Build history of the part. All positions in model axes, mm. A direction names the side the tool comes from. Give positions to 0.01 mm unless a question says otherwise; leave off trailing zeros. Loops run counter-clockwise (first coordinate to the right, second up) from the corner with the lowest first, then second, coordinate; pieces in that order, holes last.
1) Band-saw the part on C-C on y = 13.5. List the corners of the cut face in (x, z).
2) Band-saw the part on B-B on x = 1.5. List the corners of the cut face in (y, z).
3) Band-saw the part on D-D on z = 4.5. List the corners of the cut face in (x, y), then the cut area to 3 significant figures.
4) 3-axis set-ups, long thin cutter, end or side, ignore diameter. For faces 1 (the flat face through (3.81, 32.6, 6.4)), 2 (the flat face through (-3.81, 25, 6)), 3 (the flat face through (-0.1, 26.386, -3.5)): which of +Z, -Z, +X, -X, +Y, -Y reach the whole face in a straight line?
5) Band-saw the part on A-A on z = 9. List the corners of the cut face in (x, y).
6) Flat gauge pins, fed straight in: P1, Ø1, axis at y = 33, z = -5, coming from the -X side; P2, Ø6, axis at y = 6.5, z = 6.5, coming from the +X side; P3, Ø2, axis at x = 1.5, y = 27, coming from the +Z side. Where does each tip first touch, or does it go through?
7) Two-plate mould, pull along Z, no slides. Class faces 4 (the flat face through (0.04, 32.11, -5.47)), 5 (the flat face through (-2.54, 33, -5)), 6 (the cylindrical face through (-0.417, 15.653, 3.173)): +Z half, -Z half, draft (parallel to the pull), parting line (faces both ways), or undercut.
8) Wall check: line 1 (Y direction, x = 2.25, z = 4.5); line 2 (Z direction, x = 0, y = 13); line 3 (X direction, y = 11.5, z = 0). Give the ranges that are in metal, low to high.
```python
from build123d import *

# Parameters (mm, degrees)
F1_R          = 5
F2_DEPTH      = 34.64052
F3_W          = 5.08
F3_H          = 2.89434
F4_DEPTH      = 34.64052
F6_W          = 10.16
F6_H          = 5.08
F7_DEPTH      = 25.4
F8_W          = 2.54
F8_H          = 7.62
F9_DEPTH      = 3.81
F9_DEPTH_BACK = 3.81
F5_R          = 3.2004
F10_DEPTH     = 31.75
F11_R         = 0.762
F12_SIZE      = 1.27
F13_R         = 0.508


with BuildPart() as f2:
    # F1 (on Front) → F2 (new body)
    with BuildSketch(Plane.XZ):
        Circle(F1_R)
    extrude(amount=-F2_DEPTH)

    # F3 (on face) → F4 (join, through all)
    with BuildSketch(Plane.XZ):
        with Locations((0, -4.64757)):
            Rectangle(F3_W, F3_H)
    extrude(amount=-F4_DEPTH)

    # F6 (on Top) → F7 (cut)
    with BuildSketch(Plane.XY):
        with Locations((0, 28.92552)):
            Rectangle(F6_W, F6_H)
    extrude(amount=-F7_DEPTH, mode=Mode.SUBTRACT)

    # F8 (on Right) → F9 (join, two sides)
    with BuildSketch(Plane.YZ) as f9_sk:
        with Locations((32.60852, 6.35)):
            Rectangle(F8_W, F8_H)
        with Locations((24.98852, 6.35)):
            Rectangle(F8_W, F8_H)
    extrude(amount=F9_DEPTH)
    extrude(f9_sk.sketch, amount=-F9_DEPTH_BACK)

    # F5 (on face) → F10 (cut)
    with BuildSketch(Plane.XZ):
        Circle(F5_R)
    extrude(amount=-F10_DEPTH, mode=Mode.SUBTRACT)

    # F11
    f11_edges = [f2.edges().sort_by_distance(p)[0] for p in [
        (0, 26.25852, 10.16),
        (0, 31.33852, 10.16),
        (0, 33.87852, 10.16),
        (0, 23.71852, 10.16),
        (-3.81, 26.25852, 6.698943),
        (-3.81, 23.71852, 6.698943),
        (-3.81, 24.98852, 10.16),
        (-3.81, 31.33852, 6.698943),
        (-3.81, 32.60852, 10.16),
        (-3.81, 33.87852, 6.698943),
        (3.81, 24.98852, 10.16),
        (3.81, 26.25852, 6.698943),
        (3.81, 23.71852, 6.698943),
        (3.81, 31.33852, 6.698943),
        (3.81, 32.60852, 10.16),
        (3.81, 33.87852, 6.698943),
    ]]
    fillet(f11_edges, radius=F11_R)

    # F12
    f12_edges = [f2.edges().sort_by_distance(p)[0] for p in [
        (0, 26.38552, -6.09474),
        (0, 31.46552, -6.09474),
    ]]
    chamfer(f12_edges, length=F12_SIZE)

    # F13
    f13_edges = [f2.edges().sort_by_distance(p)[0] for p in [
        (-2.54, 12.55776, -6.09474),
        (-2.54, 33.68802, -6.09474),
        (2.54, 33.68802, -6.09474),
        (2.54, 12.55776, -6.09474),
    ]]
    fillet(f13_edges, radius=F13_R)


solid = f2.part
```
Findings below:
1. outline: (-2.54, -5.59) arc R0.51 ccw to (-2.03, -6.09) - (2.03, -6.09) arc R0.51 ccw to (2.54, -5.59) - (2.54, -4.31) arc R5 ccw (long way) to (-2.54, -4.31) - close; hole circle Ø6.4 at (0, 0)
2. outline: (0, -6.09) - (25.12, -6.09) - (26.39, -4.82) - (26.39, -2.83) - (0, -2.83) - close; (0, 2.83) - (31.75, 2.83) - (31.75, -2.83) - (31.47, -2.83) - (31.47, -4.82) - (32.74, -6.09) - (34.64, -6.09) - (34.64, 4.77) - (33.88, 4.77) - (33.88, 9.4) arc R0.76 ccw to (33.12, 10.16) - (32.1, 10.16) arc R0.76 ccw to (31.34, 9.4) - (31.34, 4.77) - (26.26, 4.77) - (26.26, 9.4) arc R0.76 ccw to (25.5, 10.16) - (24.48, 10.16) arc R0.76 ccw to (23.72, 9.4) - (23.72, 4.77) - (0, 4.77) - close
3. outline: (-3.81, 24.48) arc R0.76 ccw to (-3.05, 23.72) - (-2.18, 23.72) - (-2.18, 0) - (2.18, 0) - (2.18, 23.72) - (3.05, 23.72) arc R0.76 ccw to (3.81, 24.48) - (3.81, 25.5) arc R0.76 ccw to (3.05, 26.26) - (2.18, 26.26) - (2.18, 31.34) - (3.05, 31.34) arc R0.76 ccw to (3.81, 32.1) - (3.81, 33.12) arc R0.76 ccw to (3.05, 33.88) - (2.18, 33.88) - (2.18, 34.64) - (-2.18, 34.64) - (-2.18, 33.88) - (-3.05, 33.88) arc R0.76 ccw to (-3.81, 33.12) - (-3.81, 32.1) arc R0.76 ccw to (-3.05, 31.34) - (-2.18, 31.34) - (-2.18, 26.26) - (-3.05, 26.26) arc R0.76 ccw to (-3.81, 25.5) - close
3. area: 167 mm2
4. face 1: +Z, +X, +Y, -Y
4. face 2: +Z, -X, +Y, -Y
4. face 3: -Z, +X, -X
5. outline: (-3.81, 24.48) arc R0.76 ccw to (-3.05, 23.72) - (3.05, 23.72) arc R0.76 ccw to (3.81, 24.48) - (3.81, 25.5) arc R0.76 ccw to (3.05, 26.26) - (-3.05, 26.26) arc R0.76 ccw to (-3.81, 25.5) - close; (-3.81, 32.1) arc R0.76 ccw to (-3.05, 31.34) - (3.05, 31.34) arc R0.76 ccw to (3.81, 32.1) - (3.81, 33.12) arc R0.76 ccw to (3.05, 33.88) - (-3.05, 33.88) arc R0.76 ccw to (-3.81, 33.12) - close
6. P1: stops at x = -2.54
6. P2: stops at x = 3.57
6. P3: stops at z = 9.97
7. face 4: -Z half
7. face 5: draft
7. face 6: undercut
8. line 1: y = 23.72 to 26.26, 31.34 to 33.88
8. line 2: z = -6.09 to -3.2, 3.2 to 5
8. line 3: x = -5 to -3.2, 3.2 to 5
